Verification items for the finished model (mm, model axes). A direction names the side the tool comes from. Give positions to 0.01 mm unless a question says otherwise; leave off trailing zeros. Loops run counter-clockwise (first coordinate to the right, second up) from the corner with the lowest first, then second, coordinate; pieces in that order, holes last. Notation, with made-up numbers: (-35, 20.25) - (-24, 20.25) arc R29 cw to (-24, 47.25) - close; hole circle Ø4 at (56, -19). An arc over 180 degrees is marked (long way). Use one line per item in the form item = value.
```python
from build123d import *

# Parameters (mm, degrees)
F0_W     = 127
F0_H     = 107.95
F1_DEPTH = 25.4
F2_W     = 25.4
F2_H     = 19.05
F3_DEPTH = 12.7
F4_R     = 3.175
F5_R     = 1.524
F6_R     = 12.7
F7_R     = 3.175
F8_SIZE  = 0.508
F9_SIZE2 = 3.048
F9_SIZE  = 1.524


with BuildPart() as f1:
    # F0 (on Top) → F1 (new body)
    with BuildSketch(Plane.XY):
        Rectangle(F0_W, F0_H)
    extrude(amount=F1_DEPTH)

    # F2 (on face) → F3 (cut)
    with BuildSketch(Plane.XY.offset(25.4)):
        with Locations((-38.1, 31.75)):
            Rectangle(F2_W, F2_H)
    extrude(amount=-F3_DEPTH, mode=Mode.SUBTRACT)

    # F4
    f4_edges = [f1.edges().sort_by_distance(p)[0] for p in [
        (-50.8, 41.275, 19.05),
        (-50.8, 22.225, 19.05),
        (-25.4, 22.225, 19.05),
        (-25.4, 41.275, 19.05),
    ]]
    fillet(f4_edges, radius=F4_R)

    # F5
    f5_edges = [f1.edges().sort_by_distance(p)[0] for p in [
        (-38.1, 22.225, 12.7),
    ]]
    fillet(f5_edges, radius=F5_R)

    # F6
    f6_edges = [f1.edges().sort_by_distance(p)[0] for p in [
        (63.5, -53.975, 12.7),
        (63.5, 53.975, 12.7),
        (-63.5, -53.975, 12.7),
        (-63.5, 53.975, 12.7),
    ]]
    fillet(f6_edges, radius=F6_R)

    # F7
    f7_edges = [f1.edges().sort_by_distance(p)[0] for p in [
        (0, -53.975, 25.4),
    ]]
    fillet(f7_edges, radius=F7_R)

    # F8
    f8_edges = [f1.edges().sort_by_distance(p)[0] for p in [
        (0, -53.975, 0),
    ]]
    chamfer(f8_edges, length=F8_SIZE)

    # F9
    f9_edges = [f1.edges().sort_by_distance(p)[0] for p in [
        (-38.1, 41.275, 25.4),
        (-50.8, 38.1, 19.812),
        (-50.8, 31.75, 14.224),
        (-50.8, 31.75, 25.4),
        (-50.8, 25.4, 19.812),
        (-47.625, 41.275, 19.812),
        (-49.870064, 40.345064, 14.224),
        (-49.870064, 40.345064, 25.4),
        (-28.575, 41.275, 19.812),
        (-38.1, 41.275, 14.224),
        (-26.329936, 40.345064, 14.224),
        (-26.329936, 40.345064, 25.4),
        (-25.4, 38.1, 19.812),
        (-25.4, 25.4, 19.812),
        (-25.4, 31.75, 14.224),
        (-25.4, 31.75, 25.4),
        (-26.329936, 23.154936, 14.224),
        (-47.625, 22.225, 19.812),
        (-38.1, 22.225, 14.224),
        (-38.1, 22.225, 25.4),
        (-28.575, 22.225, 19.812),
        (-49.870064, 23.154936, 14.224),
        (-49.870064, 23.154936, 25.4),
    ]]
    chamfer(f9_edges, length=F9_SIZE, length2=F9_SIZE2)


solid = f1.part
```
1. Scan lines: probe 1 along X at (y, z) = (26, 16); probe 2 along X at (y, z) = (32.5, 24.25); probe 3 along Y at (x, z) = (-28, 18) (1 decimal). Record each from-to range of solid material in increasing order.
Result set:
probe_1 = -63.5 to -50.8, -25.4 to 63.5
probe_2 = -62.77 to -51.75, -24.45 to 62.77
probe_3 = -54 to 22.3, 41.2 to 54
2. Depth check by flat-ended pin: pin 1 Ø8 at (x, y) = (-36, 29.5) entering from +Z. Enter the tip coordinate at first touch or a pass-through.
Result set:
pin_1 = 12.7
3. Section check B-B, the plane x = -37. Record the cut outline in (y, z) (3 decimals), then the cut area to 3 significant figures.
Result set:
outline = (-53.975, 0.508) - (-53.467, 0) - (53.467, 0) - (53.975, 0.508) - (53.975, 22.225) arc R3.175 ccw to (50.8, 25.4) - (42.799, 25.4) - (41.275, 22.352) - (41.275, 14.224) arc R1.524 cw to (39.751, 12.7) - (23.749, 12.7) arc R1.524 cw to (22.225, 14.224) - (22.225, 22.352) - (20.701, 25.4) - (-50.8, 25.4) arc R3.175 ccw to (-53.975, 22.225) - close
area = 2,490 mm²
4. Section check A-A, the plane z = 18. Record the cut outline in (x, y) (3 decimals), then the cut area to 3 significant figures.
Result set:
outline = (-63.5, -41.275) arc R12.7 ccw to (-50.8, -53.975) - (50.8, -53.975) arc R12.7 ccw to (63.5, -41.275) - (63.5, 41.275) arc R12.7 ccw to (50.8, 53.975) - (-50.8, 53.975) arc R12.7 ccw to (-63.5, 41.275) - close; hole (-50.8, 25.4) arc R3.175 ccw to (-47.625, 22.225) - (-28.575, 22.225) arc R3.175 ccw to (-25.4, 25.4) - (-25.4, 38.1) arc R3.175 ccw to (-28.575, 41.275) - (-47.625, 41.275) arc R3.175 ccw to (-50.8, 38.1) - close
area = 13,100 mm²
5. Tool access check on faces 5 (the flat face through (-25.4, 32, 18)), 6 (the cylindrical face through (59.681, -50.353, 11.519)). Record the directions out of +Z, -Z, +X, -X, +Y, -Y that give a thin tool (end or side, any length) a straight path to the whole face; none if there is none.
Result set:
face_5 = +Z
face_6 = +Z, -Z, +X, -Y
6. Draft check along X on faces 1 (the flat face through (-38, 41.275, 18)), 2 (the cylindrical face through (-26.305, 40.32, 18.231)), 3 (the flat face through (-1, -53.975, 11)), 4 (the flat face through (63.5, -1, 11)). Enter one of: released by +X, released by -X, zero draft, split by the parting line, or undercut.
Result set:
face_1 = undercut
face_2 = undercut
face_3 = zero draft
face_4 = released by +X
